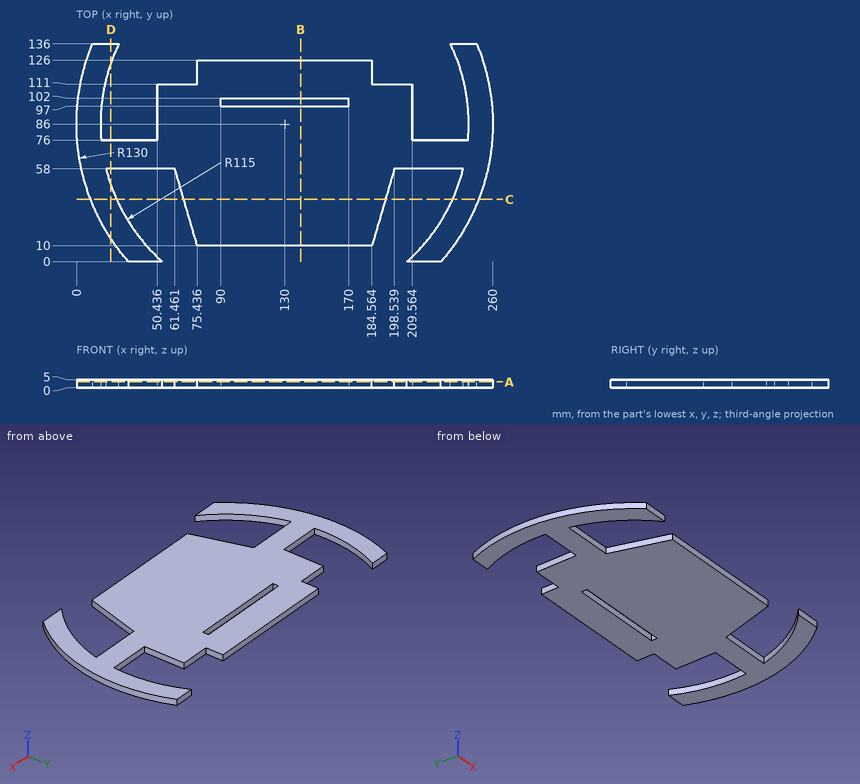
Design review of the part shown in the three views and the two pictorial views. Dimensions are in mm from the part's minimum x, y and z. Round coordinates to 2 decimals unless told otherwise and drop trailing zeros. Order: outer loops, then holes, each group sorted by start corner. A loop starts at its lowest first (then second) coordinate and runs counter-clockwise, first axis right, second up.
Q1. Insertion check: P1, Ø2.5, axis at x = 116.5, z = 3, coming from the -Y side; P2, Ø1.5, axis at y = 98.5, z = 1.5, coming from the -X side; P3, Ø1.5, axis at x = 126, z = 3, coming from the +Y side; P4, Ø3, axis at x = 122, y = 76, coming from the -Z side. Each pin has a flat end and moves straight along its axis. Give the tip position at first contact, or say it passes through.
Findings below:
P1: stops at y = 10
P2: stops at x = 0.53
P3: stops at y = 126
P4: stops at z = 0
Q2. We need section D-D, the plane x = 21.5. Give the boundary of the cut face in (y, z) (1 decimal).
Findings below:
outline: (14.4, 0) - (47.9, 0) - (47.9, 5) - (14.4, 5) - close; (58, 0) - (76, 0) - (76, 5) - (58, 5) - close; (124.1, 0) - (136, 0) - (136, 5) - (124.1, 5) - close
Q3. Wall thickness on line 1 (Y direction, x = 92, z = 1.25); line 2 (X direction, y = 43, z = 2.45); line 3 (X direction, y = 103.5, z = 4.6) (1 decimal): over which ranges is each line inside the solid? List them lowest first.
Findings below:
line 1: y = 10 to 97, 102 to 126
line 2: x = 7.32 to 23.34, 65.83 to 194.17, 236.66 to 252.68
line 3: x = 1.2 to 16.3, 50.4 to 209.6, 243.7 to 258.8
Q4. We need section C-C, the plane y = 39. Give the boundary of the cut face in (x, z).
Findings below:
outline: (8.79, 0) - (25.04, 0) - (25.04, 5) - (8.79, 5) - close; (66.99, 0) - (193.01, 0) - (193.01, 5) - (66.99, 5) - close; (234.96, 0) - (251.21, 0) - (251.21, 5) - (234.96, 5) - close
Q5. We need section A-A, the plane z = 3.65. Give the boundary of the cut face in (x, y) (1 decimal).
Findings below:
outline: (10, 136) arc R130 ccw to (32.5, 0) - (53.7, 0) arc R115 cw to (18.5, 58) - (61.5, 58) - (75.4, 10) - (184.6, 10) - (198.5, 58) - (241.5, 58) arc R115 cw to (206.3, 0) - (227.5, 0) arc R130 ccw to (250, 136) - (233.6, 136) arc R115 cw to (244.6, 76) - (209.6, 76) - (209.6, 111) - (184.6, 111) - (184.6, 126) - (75.4, 126) - (75.4, 111) - (50.4, 111) - (50.4, 76) - (15.4, 76) arc R115 cw to (26.4, 136) - close; hole (90, 97) - (170, 97) - (170, 102) - (90, 102) - close
Q6. We need section B-B, the plane x = 140. Give the boundary of the cut face in (y, z).
Findings below:
outline: (10, 0) - (97, 0) - (97, 5) - (10, 5) - close; (102, 0) - (126, 0) - (126, 5) - (102, 5) - close
